Input: part model. Units: mm. Frame: model coordinates. A direction names the side the tool comes from. Give positions to 0.01 mm unless a question says otherwise; leave off trailing zeros. Write each loop counter-clockwise with the first axis right and the second up, starting at its lowest first coordinate (ties: lowest second). Pieces come first, ordered by that corner, then holes.
```python
from build123d import *

# Parameters (mm, degrees)
F1_W        = 60
F1_H        = 93
F2_DEPTH    = 8
F3_T1_DEPTH = 147.142599219
F4_T1_DEPTH = 102.8305675527
F5_DEPTH    = 25
F6_DEPTH    = 6
F7_T1_DEPTH = 105.1482614058


# Not quite as in the source:
# - a fillet or chamfer that OpenCascade refuses, or shapes differently, is made with other operations: its cross-section is extruded or revolved along the edge and cut away or added


with BuildPart() as f2:
    # F1 (on Top) → F2 (new body)
    with BuildSketch(Plane.XY):
        Rectangle(F1_W, F1_H)
    extrude(amount=F2_DEPTH)

    # F3: chamfer of 4.325 x 10.4414736573 on 2 edges, made by hand

    # F3_s2 → F3_t1 (cut)
    with BuildSketch(Plane.XZ.offset(-73.5712996095)):
        Polygon((30, -2.4414736573), (25.675, 8), (30, 8), align=None)
        Polygon((-30, -2.4414736573), (-25.675, 8), (-30, 8), align=None)
    extrude(amount=F3_T1_DEPTH, mode=Mode.SUBTRACT)

    # F4: chamfer of 9 x 9.9955126335 on 1 edges, made by hand

    # F4_s2 → F4_t1 (cut)
    with BuildSketch(Plane.YZ.offset(-51.4152837764)):
        Polygon((37.5, 8), (46.5, -1.9955126335), (46.5, 8), align=None)
    extrude(amount=F4_T1_DEPTH, mode=Mode.SUBTRACT)

    # F0 (on Top) → F5 (cut)
    with BuildSketch(Plane.XY):
        with BuildLine():
            ThreePointArc((23, 24.5), (21.8284271247, 27.3284271247), (19, 28.5))
            Line((19, 28.5), (-19, 28.5))
            ThreePointArc((-19, 28.5), (-21.8284271247, 27.3284271247), (-23, 24.5))
            Line((-23, 24.5), (-23, -24.5))
            ThreePointArc((-23, -24.5), (-21.8284271247, -27.3284271247), (-19, -28.5))
            Line((-19, -28.5), (19, -28.5))
            ThreePointArc((19, -28.5), (21.8284271247, -27.3284271247), (23, -24.5))
            Line((23, -24.5), (23, 24.5))
        make_face()
    extrude(amount=F5_DEPTH, mode=Mode.SUBTRACT)

    # F0 (on Top) → F6 (cut)
    with BuildSketch(Plane.XY):
        with BuildLine():
            ThreePointArc((25.6034387499, 30.25), (25.0176523123, 31.6642135624), (23.6034387499, 32.25))
            Line((23.6034387499, 32.25), (-23.3965612501, 32.25))
            ThreePointArc((-23.3965612501, 32.25), (-24.8107748125, 31.6642135624), (-25.3965612501, 30.25))
            Line((-25.3965612501, 30.25), (-25.3965612501, -35.75))
            ThreePointArc((-25.3965612501, -35.75), (-24.8107748125, -37.1642135624), (-23.3965612501, -37.75))
            Line((-23.3965612501, -37.75), (23.6034387499, -37.75))
            ThreePointArc((23.6034387499, -37.75), (25.0176523123, -37.1642135624), (25.6034387499, -35.75))
            Line((25.6034387499, -35.75), (25.6034387499, 30.25))
        make_face()
        with BuildLine():
            Line((-19, 28.5), (19, 28.5))
            ThreePointArc((19, 28.5), (21.8284271247, 27.3284271247), (23, 24.5))
            Line((23, 24.5), (23, -24.5))
            ThreePointArc((23, -24.5), (21.8284271247, -27.3284271247), (19, -28.5))
            Line((19, -28.5), (-19, -28.5))
            ThreePointArc((-19, -28.5), (-21.8284271247, -27.3284271247), (-23, -24.5))
            Line((-23, -24.5), (-23, 24.5))
            ThreePointArc((-23, 24.5), (-21.8284271247, 27.3284271247), (-19, 28.5))
        make_face(mode=Mode.SUBTRACT)
    extrude(amount=F6_DEPTH, mode=Mode.SUBTRACT)

    # F7: chamfer of 8 x 10.4258029827 on 1 edges, made by hand

    # F7_s2 → F7_t1 (cut)
    with BuildSketch(Plane.YZ.offset(-52.5741307029)):
        Polygon((-46.5, -2.4258029827), (-38.5, 8), (-46.5, 8), align=None)
    extrude(amount=F7_T1_DEPTH, mode=Mode.SUBTRACT)


solid = f2.part
```
Q1. Section B-B, the plane x = 3. Return the cut outline in (y, z).
Q2. Section D-D, the plane y = -32. Return the cut outline in (x, z) (3 decimals).
Q3. Pin query (flat end, axial travel): pin 1 (3 mm diameter, centred on x = -20, y = 30, fed in from -Z); pin 2 (2 mm diameter, centred on y = 8, z = 2, fed in from +X); pin 3 (1.8 mm diameter, centred on y = -13, z = 4, fed in from +X). Return the tip coordinate at first contact, or that it passes through.
Q4. Material intervals for line 1 along Z through (x, y) = (25, 25); line 2 along X through (y, z) = (-28, 4.75); line 3 along Y through (x, z) = (11.5, 5.75), sorted ascending.
Q5. Section C-C, the plane z = 3. Return the cut outline in (x, y).
Q6. Mould query, pull axis Y, two halves, no side actions, for faces 4 (the cylindrical face through (-21.797, 27.359, 6.986)), 5 (the flat face through (-0.406, -41.612, 3.944)), 6 (the flat face through (27.355, 0.658, 3.944)), 7 (the cylindrical face through (-21.859, -27.297, 6.986)). Classes: +Y half, -Y half, draft (parallel to the pull), parting line (faces both ways), or undercut.
Q7. Section A-A, the plane y = -8.5. Return the cut outline in (x, z) (3 decimals), then the cut area to 3 significant figures.
Q8. Access query for faces 1 (the flat face through (23, 0, 7)), 2 (the cylindrical face through (25.03, 31.65, 2.96)), 3 (the flat face through (-27.355, 0.658, 3.944)). Directions: +Z, -Z, +X, -X, +Y, -Y. A direction counts if a zero-diameter tool reaches every point of the face in a straight line with its end or side. Return the directions, or none.
Solutions:
1. outline: (-44.64, 0) - (-37.75, 0) - (-37.75, 6) - (-28.5, 6) - (-28.5, 8) - (-38.5, 8) - close; (28.5, 6) - (32.25, 6) - (32.25, 0) - (44.7, 0) - (37.5, 8) - (28.5, 8) - close
2. outline: (-28.989, 0) - (-25.397, 0) - (-25.397, 6) - (25.603, 6) - (25.603, 0) - (28.989, 0) - (25.675, 8) - (-25.675, 8) - close
3. pin 1: stops at z = 6
3. pin 2: stops at x = 28.57
3. pin 3: stops at x = 27.7
4. line 1: z = 6 to 8
4. line 2: x = -27.02 to -25.4, 25.6 to 27.02
4. line 3: y = -40.23 to -37.75, 32.25 to 39.53
5. outline: (-27.75, -42.34) - (27.75, -42.34) - (27.75, 42) - (-27.75, 42) - close; hole (-25.4, -35.75) arc R2 ccw to (-23.4, -37.75) - (23.6, -37.75) arc R2 ccw to (25.6, -35.75) - (25.6, 30.25) arc R2 ccw to (23.6, 32.25) - (-23.4, 32.25) arc R2 ccw to (-25.4, 30.25) - close
6. face 4: undercut
6. face 5: -Y half
6. face 6: draft
6. face 7: undercut
7. outline: (-28.989, 0) - (-25.397, 0) - (-25.397, 6) - (-23, 6) - (-23, 8) - (-25.675, 8) - close; (23, 6) - (25.603, 6) - (25.603, 0) - (28.989, 0) - (25.675, 8) - (23, 8) - close
7. area: 39.3 mm2
8. face 1: +Z, -Z
8. face 2: -Z
8. face 3: +Z, -X, +Y, -Y
